Here's how the part is built. I have some questions about the finished solid (model axes, mm). Give positions to 0.01 mm unless a question says otherwise; leave off trailing zeros. Loops run counter-clockwise (first coordinate to the right, second up) from the corner with the lowest first, then second, coordinate; pieces in that order, holes last.
Q1. If we section it at A-A (y = -25.5): Please give me the cut outline in (x, z).
Q2. If we section it at C-C (x = 72.5): Please give me the cut outline in (y, z).
Q3. If we section it at B-B (z = 11): Please give me the cut outline in (x, y), plus the area to 3 significant figures.
Q4. I need wall thicknesses on line 1 (Y direction, x = 33.5, z = 43.5); line 2 (Y direction, x = -74, z = 87); line 3 (X direction, y = -21.5, z = 84). Which ranges of each line are inside material? Lowest first, please.
Q5. Will these pins go through, and if not, where does the flat tip stop? P1, Ø1.5, axis at x = -58.5, z = 12, coming from the +Y side; P2, Ø2, axis at y = -20.5, z = 14.5, coming from the +X side; P3, Ø8, axis at y = 30.5, z = 11.5, coming from the +X side.
from build123d import *

# Parameters (mm, degrees)
F0_R      = 93.952715
F1_DEPTH  = 381
F1_FACE_R = 93.952715
F2_DEPTH  = 76.2
F3_R      = 89.547505
F4_DEPTH  = 100.42847


with BuildPart() as f1:
    # F0 (on Top) → F1 (new body)
    with BuildSketch(Plane.XY):
        Circle(F0_R)
    extrude(amount=F1_DEPTH)

    # F1_face (on face) → F2 (cut)
    with BuildSketch(Plane.XY.offset(381)):
        Circle(F1_FACE_R)
    extrude(amount=-F2_DEPTH, mode=Mode.SUBTRACT)

    # F3 (on face) → F4 (intersect)
    with BuildSketch(Plane(origin=(0, 0, 0), x_dir=(1, 0, 0), z_dir=(0, 0, -1))):
        Circle(F3_R)
    extrude(amount=-F4_DEPTH, mode=Mode.INTERSECT)


solid = f1.part
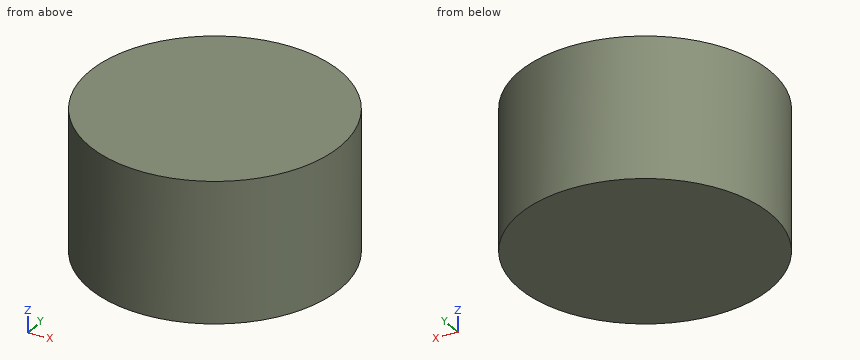
Check sheet entries:
1. outline: (-85.84, 0) - (85.84, 0) - (85.84, 100.43) - (-85.84, 100.43) - close
2. outline: (-52.56, 0) - (52.56, 0) - (52.56, 100.43) - (-52.56, 100.43) - close
3. outline: circle Ø179.1 at (0, 0)
3. area: 25,200 mm2
4. line 1: y = -83.05 to 83.05
4. line 2: y = -50.43 to 50.43
4. line 3: x = -86.93 to 86.93
5. P1: stops at y = 68.44
5. P2: stops at x = 87.4
5. P3: stops at x = 85.54
